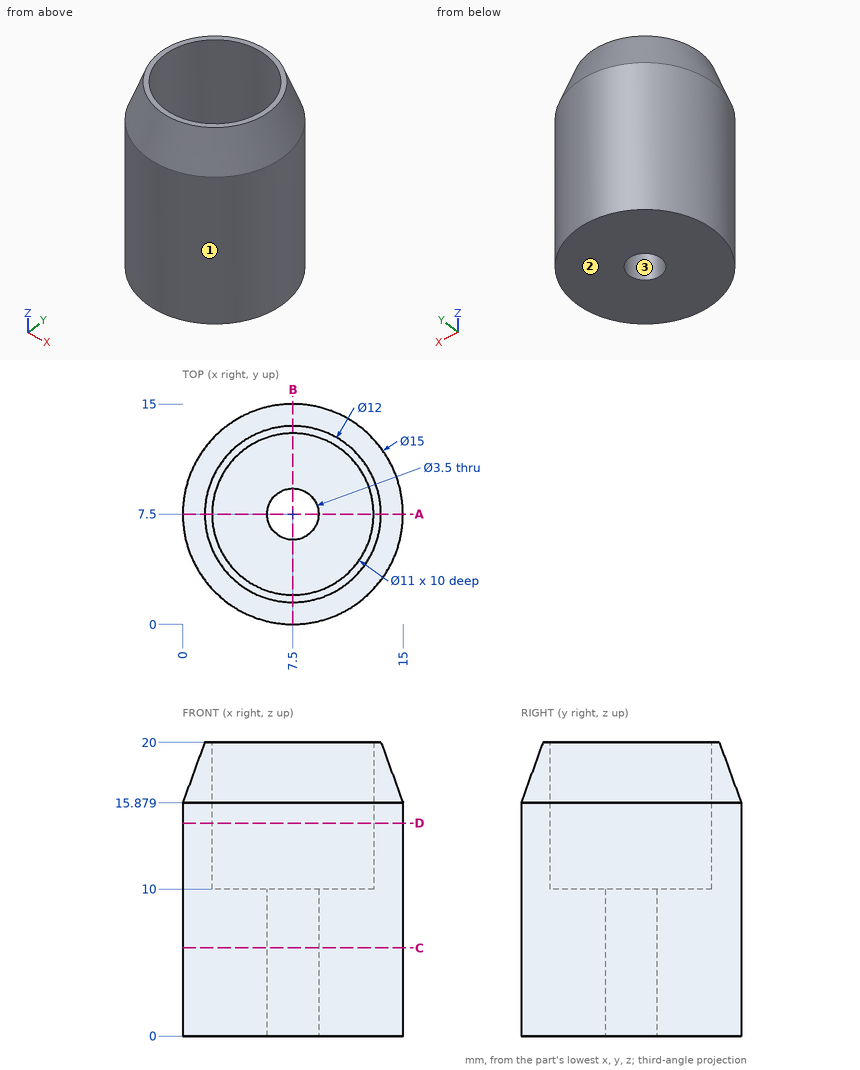
Geometry: see drawing. Coordinates: mm, zero at the bounding-box minimum. Coordinates: 2 decimals unless noted, no trailing zeros. Loops run counter-clockwise (first coordinate to the right, second up) from the corner with the lowest first, then second, coordinate; pieces in that order, holes last.
(1) First-contact query: pin 1 Ø3 at (x, z) = (12.5, 11) entering from +Y; pin 2 Ø4.5 at (x, y) = (7.5, 7.5) entering from +Z; pin 3 Ø4 at (x, y) = (3.5, 7) entering from -Z; pin 4 Ø1.5 at (y, z) = (8.5, 10) entering from -X. Flat tips, straight axial feed; report the tip coordinate or a pass-through.
(2) Material intervals for probe 1 along Y at (x, z) = (7.5, 13.75); probe 2 along Y at (x, z) = (7.5, 7); probe 3 along Z at (x, y) = (3.5, 9), sorted ascending.
(3) Section A-A on y = 7.5. Return the cut outline in (x, z), then the cut area to 3 significant figures.
(4) Section D-D on z = 14.5. Return the cut outline in (x, y).
(5) Section C-C on z = 6. Return the cut outline in (x, y).
(6) Pull-direction query (Y, two-part tool) for the marked faces 1, 2 and 3; classes: released by +Y, released by -Y, zero draft, split by the parting line, or undercut.
Data:
1. pin 1: stops at y = 14.13
1. pin 2: stops at z = 10
1. pin 3: stops at z = 0
1. pin 4: stops at x = 0
2. probe 1: y = 0 to 2, 13 to 15
2. probe 2: y = 0 to 5.75, 9.25 to 15
2. probe 3: z = 0 to 10
3. outline: (0, 0) - (5.75, 0) - (5.75, 10) - (2, 10) - (2, 20) - (1.5, 20) - (0, 15.88) - close; (9.25, 0) - (15, 0) - (15, 15.88) - (13.5, 20) - (13, 20) - (13, 10) - (9.25, 10) - close
3. area: 149 mm2
4. outline: circle Ø15 at (7.5, 7.5); hole circle Ø11 at (7.5, 7.5)
5. outline: circle Ø15 at (7.5, 7.5); hole circle Ø3.5 at (7.5, 7.5)
6. face 1: split by the parting line
6. face 2: zero draft
6. face 3: undercut
